For this review, take the finished solid that the model builds, in its own axes (mm). Face numbers are marked on the shaded views. A direction names the side the tool comes from. Round coordinates to 2 decimals unless told otherwise and drop trailing zeros. Order: outer loops, then holes, each group sorted by start corner. A loop starts at its lowest first (then second) coordinate and runs counter-clockwise, first axis right, second up. Notation, with made-up numbers: M -24.75,-6.75 L 17.25,-6.75 A18 ccw 17.25,14.25 Z; hole C -28,83 d2. An arc over 180 degrees is marked long. Put each result on its own line as item: value.
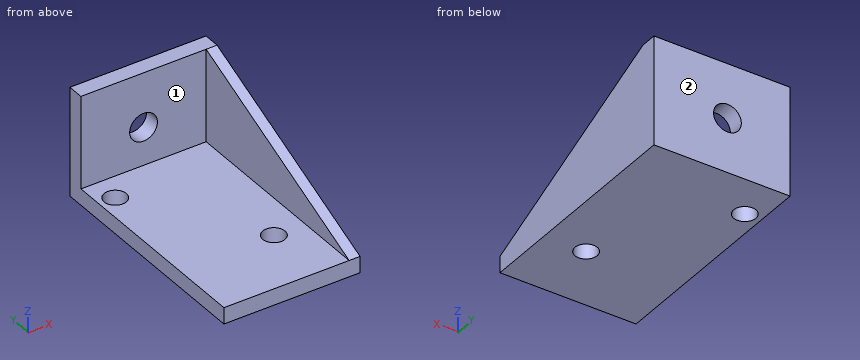
from build123d import *

# Parameters (mm, degrees)
SKETCH1_W           = 23
SKETCH1_H           = 42.000000074
SKETCH1_R           = 2.05
BOSS_EXTRUDE1_DEPTH = 3
SKETCH2_W           = 23
SKETCH2_H           = 17
SKETCH2_R           = 2.55
BOSS_EXTRUDE2_DEPTH = 3
BOSS_EXTRUDE3_DEPTH = 2


with BuildPart() as part:
    # Sketch1 → Boss-Extrude1 (new body)
    with BuildSketch(Plane.XY):
        with Locations((11.5, 21.000000037)):
            Rectangle(SKETCH1_W, SKETCH1_H)
        with Locations((17.34, 12.13)):
            Circle(SKETCH1_R, mode=Mode.SUBTRACT)
        with Locations((2.99, 34.1)):
            Circle(SKETCH1_R, mode=Mode.SUBTRACT)
    extrude(amount=BOSS_EXTRUDE1_DEPTH)

    # Sketch2 → Boss-Extrude2 (add)
    with BuildSketch(Plane(origin=(0, 42.000000074, 0), x_dir=(1, 0, 0), z_dir=(0, 1, 0))):
        with Locations((11.5, -11.5)):
            Rectangle(SKETCH2_W, SKETCH2_H)
        with Locations((11.5, -10)):
            Circle(SKETCH2_R, mode=Mode.SUBTRACT)
    extrude(amount=-BOSS_EXTRUDE2_DEPTH)

    # Sketch3 → Boss-Extrude3 (add)
    with BuildSketch(Plane(origin=(23, 0, 0), x_dir=(0, 0, -1), z_dir=(1, 0, 0))):
        Polygon((-20, 39.000000074), (-3, 0), (0, 0), (0, 42.000000074), (-20, 42.000000074), align=None)
    extrude(amount=BOSS_EXTRUDE3_DEPTH)


solid = part.part
(1) Add section A-A on x = 11.5. Give the boundary of the cut face in (y, z), then the cut area to 3 significant figures.
A:
outline: M 0,0 L 42,0 L 42,7.45 L 39,7.45 L 39,3 L 0,3 Z; M 39,12.55 L 42,12.55 L 42,20 L 39,20 Z
area: 162 mm2
(2) To check wall thickness, follow L1, parallel to Z at x = 11.5, y = 40.5; L2, parallel to Y at x = 2.99, z = 2; L3, parallel to X at y = 39.8, z = 10. State the ranges of each line that lie inside material, in increasing order.
A:
L1: z = 0 to 7.45, 12.55 to 20
L2: y = 0 to 32.05, 36.15 to 42
L3: x = 0 to 8.95, 14.05 to 25
(3) Add section B-B on y = 35. Give the boundary of the cut face in (x, z).
A:
outline: M 0,0 L 1.15,0 L 1.15,3 L 0,3 Z; M 4.83,0 L 25,0 L 25,18.26 L 23,18.26 L 23,3 L 4.83,3 Z
(4) Add section C-C on x = 5.75. Give the boundary of the cut face in (y, z), then the cut area to 3 significant figures.
A:
outline: M 0,0 L 42,0 L 42,20 L 39,20 L 39,3 L 0,3 Z
area: 177 mm2
(5) For the marked faces 1 and 2, list the 3-axis set-ups (+Z, -Z, +X, -X, +Y, -Y) from which the entire face can be reached by the end or side of a thin tool; tool diameter is ignored.
A:
face 1: +Z, -X, -Y
face 2: +Z, -Z, +X, -X, +Y
(6) Insertion check: pin 1 Ø1.5 at (x, z) = (20, 10.5) entering from -Y; pin 2 Ø8 at (x, y) = (6, 28) entering from +Z. Each pin has a flat end and moves straight along its axis. Give the tip position at first contact, or say it passes through.
A:
pin 1: stops at y = 39
pin 2: stops at z = 3
(7) Add section D-D on z = 6.5. Give the boundary of the cut face in (x, y).
A:
outline: M 0,39 L 23,39 L 23,8.03 L 25,8.03 L 25,42 L 0,42 Z
